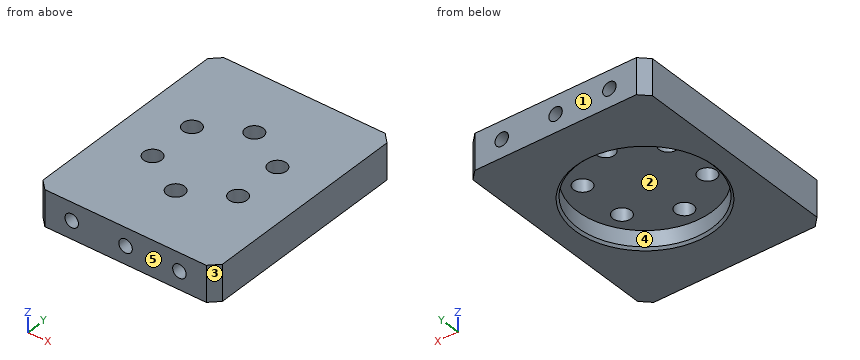
from build123d import *

# Parameters (mm, degrees)
SKETCH_1_W          = 40
SKETCH_1_H          = 50
EXTRUDE_1_DEPTH     = 8
SKETCH_2_R          = 15
CUT_EXTRUDE_1_DEPTH = 4
SKETCH_3_R          = 2
CUT_EXTRUDE_2_DEPTH = 10
CHAMFER_1_SIZE      = 2
SKETCH_4_R          = 1.5
CUT_EXTRUDE_3_DEPTH = 6
CUT_EXTRUDE_START   = -6
SKETCH_5_R          = 1.5
CUT_EXTRUDE_4_DEPTH = 6
CHAMFER_2_SIZE      = 0.5


with BuildPart() as part:
    # 草图1 → 凸台-拉伸1 (new body)
    with BuildSketch(Plane.XY):
        Rectangle(SKETCH_1_W, SKETCH_1_H)
    extrude(amount=EXTRUDE_1_DEPTH)

    # 草图2 → 切除-拉伸1 (cut)
    with BuildSketch(Plane(origin=(0, 0, 0), x_dir=(-1, 0, 0), z_dir=(0, 0, -1))):
        Circle(SKETCH_2_R)
    extrude(amount=-CUT_EXTRUDE_1_DEPTH, mode=Mode.SUBTRACT)

    # 草图3 → 切除-拉伸2 (cut)
    with BuildSketch(Plane(origin=(0, 0, 4), x_dir=(-1, 0, 0), z_dir=(0, 0, -1))):
        with Locations((0, 11)):
            Circle(SKETCH_3_R)
        with Locations((9.526279442, 5.5)):
            Circle(SKETCH_3_R)
        with Locations((9.526279442, -5.5)):
            Circle(SKETCH_3_R)
        with Locations((0, -11)):
            Circle(SKETCH_3_R)
        with Locations((-9.526279442, -5.5)):
            Circle(SKETCH_3_R)
        with Locations((-9.526279442, 5.5)):
            Circle(SKETCH_3_R)
    extrude(amount=-CUT_EXTRUDE_2_DEPTH, mode=Mode.SUBTRACT)

    # 倒角1
    chamfer_1_edges = [part.edges().sort_by_distance(p)[0] for p in [
        (20, -25, 4),
        (-20, -25, 4),
        (-20, 25, 4),
        (20, 25, 4),
    ]]
    chamfer(chamfer_1_edges, length=CHAMFER_1_SIZE)

    # 草图4 → 切除-拉伸3 (cut)
    with BuildSketch(Plane(origin=(0, 25, 0), x_dir=(1, 0, 0), z_dir=(0, 1, 0))):
        with Locations(Location((-12, -4, 0), (0, 0, 270))):
            Circle(SKETCH_4_R)
        with Locations(Location((0, -4, 0), (0, 0, 270))):
            Circle(SKETCH_4_R)
        with Locations(Location((12, -4, 0), (0, 0, 270))):
            Circle(SKETCH_4_R)
    extrude(amount=-CUT_EXTRUDE_3_DEPTH, mode=Mode.SUBTRACT)

    # 草图5 → 切除-拉伸4 (cut)
    with BuildSketch(Plane.XZ.offset(25).offset(CUT_EXTRUDE_START)):
        with Locations(Location((-12, 4, 0), (0, 0, 90))):
            Circle(SKETCH_5_R)
        with Locations(Location((0, 4, 0), (0, 0, 90))):
            Circle(SKETCH_5_R)
        with Locations(Location((12, 4, 0), (0, 0, 90))):
            Circle(SKETCH_5_R)
    extrude(amount=CUT_EXTRUDE_4_DEPTH, mode=Mode.SUBTRACT)

    # 倒角2
    chamfer_2_edges = [part.edges().sort_by_distance(p)[0] for p in [
        (15, 0, 0),
    ]]
    chamfer(chamfer_2_edges, length=CHAMFER_2_SIZE)


solid = part.part
Read the model definition and answer for the solid it produces. Units are mm, in the model's axes. Face numbers are marked on the shaded views. A direction names the side the tool comes from. Round coordinates to 2 decimals unless told otherwise and drop trailing zeros. Write each loop counter-clockwise with the first axis right and the second up, starting at its lowest first coordinate (ties: lowest second). Pieces come first, ordered by that corner, then holes.
1. Given pin 1 Ø1.8 at (x, z) = (12, 4) entering from -Y; pin 2 Ø3 at (x, y) = (-9.53, -5.5) entering from -Z; pin 3 Ø6.5 at (x, y) = (9.53, 5.5) entering from -Z, each flat-ended and moving along its own axis, determine where each tip first touches the part or whether it passes through.
2. Which of the six approach directions +Z, -Z, +X, -X, +Y, -Y give full straight-line access (tool end or side, diameter ignored) to the marked faces 4 and 5?
3. Straight lines are drawn through the part: L1, parallel to Y at x = -9.5, z = 6; L2, parallel to X at y = -20.45, z = 4; L3, parallel to X at y = -23, z = 3. For each, find the intervals that lie inside material, in ascending order.
4. Determine the mould class of the marked faces 1, 2 and 3 for opening direction Y: pulls with the +Y half, pulls with the -Y half, needs draft (parallel to the pull), parting line crosses it, or undercut.
5. The part is cut by section A-A, the plane x = 0. Determine the outline of the cut face in (y, z).
6. The part is cut by section D-D, the plane x = 9.5. State how many separate pieces and enclosed holes the cut face has, then the cut area to 3 significant figures.
7. The part is cut by section B-B, the plane z = 7.25. Determine the outline of the cut face in (x, y).
8. The part is cut by section C-C, the plane y = 0. Determine the outline of the cut face in (x, z), then the cut area to 3 significant figures.
Values:
1. pin 1: stops at y = -19
1. pin 2: passes through
1. pin 3: stops at z = 4
2. face 4: -Z
2. face 5: +Z, -Z, +X, -X, -Y
3. L1: y = -25 to -7.5, -3.5 to 3.5, 7.5 to 25
3. L2: x = -20 to -13.5, -10.5 to -1.5, 1.5 to 10.5, 13.5 to 20
3. L3: x = -20 to -13.12, -10.88 to -1.12, 1.12 to 10.88, 13.12 to 20
4. face 1: pulls with the +Y half
4. face 2: undercut
4. face 3: pulls with the -Y half
5. outline: (-25, 0) - (-15.5, 0) - (-15, 0.5) - (-15, 4) - (-13, 4) - (-13, 8) - (-25, 8) - (-25, 5.5) - (-19, 5.5) - (-19, 2.5) - (-25, 2.5) - close; (-9, 4) - (9, 4) - (9, 8) - (-9, 8) - close; (13, 4) - (15, 4) - (15, 0.5) - (15.5, 0) - (25, 0) - (25, 2.5) - (19, 2.5) - (19, 5.5) - (25, 5.5) - (25, 8) - (13, 8) - close
6. separate pieces: 3
6. enclosed holes: 0
6. area: 275 mm2
7. outline: (-20, -23) - (-18, -25) - (18, -25) - (20, -23) - (20, 23) - (18, 25) - (-18, 25) - (-20, 23) - close; hole circle Ø4 at (-9.53, -5.5); hole circle Ø4 at (-9.53, 5.5); hole circle Ø4 at (0, -11); hole circle Ø4 at (0, 11); hole circle Ø4 at (9.53, -5.5); hole circle Ø4 at (9.53, 5.5)
8. outline: (-20, 0) - (-15.5, 0) - (-15, 0.5) - (-15, 4) - (15, 4) - (15, 0.5) - (15.5, 0) - (20, 0) - (20, 8) - (-20, 8) - close
8. area: 200 mm2
